Read the model definition and answer for the solid it produces. Units are mm, in the model's axes. A direction names the side the tool comes from. Give positions to 0.01 mm unless a question says otherwise; leave off trailing zeros. Order: outer loops, then holes, each group sorted by start corner. A loop starts at its lowest first (then second) coordinate and runs counter-clockwise, first axis right, second up. Notation, with made-up numbers: M 88,49.5 L 98,49.5 A13 cw 98,59.5 Z; hole C -37.75,63 d9. An arc over 180 degrees is marked long. One line per item, written item: value.
from build123d import *

# Parameters (mm, degrees)
PANEL_W                      = 1000
PANEL_H                      = 300
PANEL_R                      = 117.475
PANEL_R_2                    = 38
PANEL_PLY_DEPTH              = 12
PIZEO_POCKET_CUT_DEPTH       = 3
SKETCH6_R                    = 15
CORD_CUT_DEPTH               = 12
SKETCH7_W                    = 1000
SKETCH7_H                    = 12
HORIZONTAL_HOUSING_CUT_DEPTH = 4
SKETCH8_W                    = 12
SKETCH8_H                    = 276
VERTICAL_HOUSING_CUT_DEPTH   = 4
SKETCH9_R                    = 128.5875
CUT_EXTRUDE1_DEPTH           = 1


with BuildPart() as part:
    # Panel → Panel Ply (new body)
    with BuildSketch(Plane.XY):
        with Locations((500, 150)):
            Rectangle(PANEL_W, PANEL_H)
        with Locations((242, 150)):
            Circle(PANEL_R, mode=Mode.SUBTRACT)
        with Locations((758, 150)):
            Circle(PANEL_R, mode=Mode.SUBTRACT)
        with Locations((68, 150)):
            Circle(PANEL_R_2, mode=Mode.SUBTRACT)
        with Locations(Location((932, 150, 0), (0, 0, 180))):
            Circle(PANEL_R_2, mode=Mode.SUBTRACT)
    extrude(amount=PANEL_PLY_DEPTH)

    # Sketch4 → Pizeo Pocket Cut (cut)
    with BuildSketch(Plane.XY.offset(12)):
        with BuildLine():
            Line((32, 194), (104, 194))
            ThreePointArc((104, 194), (109.656854249, 191.656854249), (112, 186))
            Line((112, 186), (112, 114))
            ThreePointArc((112, 114), (109.656854249, 108.343145751), (104, 106))
            Line((104, 106), (32, 106))
            ThreePointArc((32, 106), (26.343145751, 108.343145751), (24, 114))
            Line((24, 114), (24, 186))
            ThreePointArc((24, 186), (26.343145751, 191.656854249), (32, 194))
        make_face()
        with BuildLine():
            Line((968, 106), (896, 106))
            ThreePointArc((896, 106), (890.343145751, 108.343145751), (888, 114))
            Line((888, 114), (888, 186))
            ThreePointArc((888, 186), (890.343145751, 191.656854249), (896, 194))
            Line((896, 194), (968, 194))
            ThreePointArc((968, 194), (973.656854249, 191.656854249), (976, 186))
            Line((976, 186), (976, 114))
            ThreePointArc((976, 114), (973.656854249, 108.343145751), (968, 106))
        make_face()
    extrude(amount=-PIZEO_POCKET_CUT_DEPTH, mode=Mode.SUBTRACT)

    # Sketch6 → Cord Cut (cut)
    with BuildSketch(Plane.XY.offset(12)):
        with Locations((500, 255)):
            Circle(SKETCH6_R)
    extrude(amount=-CORD_CUT_DEPTH, mode=Mode.SUBTRACT)

    # Sketch7 → Horizontal Housing Cut (cut)
    with BuildSketch(Plane.XY.offset(12)):
        with Locations((500, 294)):
            Rectangle(SKETCH7_W, SKETCH7_H)
        with Locations((500, 6)):
            Rectangle(SKETCH7_W, SKETCH7_H)
    extrude(amount=-HORIZONTAL_HOUSING_CUT_DEPTH, mode=Mode.SUBTRACT)

    # Sketch8 → Vertical Housing Cut (cut)
    with BuildSketch(Plane.XY.offset(12)):
        with Locations((6, 150)):
            Rectangle(SKETCH8_W, SKETCH8_H)
        with Locations((994, 150)):
            Rectangle(SKETCH8_W, SKETCH8_H)
        with Locations((411, 150)):
            Rectangle(SKETCH8_W, SKETCH8_H)
        with Locations((589, 150)):
            Rectangle(SKETCH8_W, SKETCH8_H)
    extrude(amount=-VERTICAL_HOUSING_CUT_DEPTH, mode=Mode.SUBTRACT)

    # Sketch9 → Cut-Extrude1 (cut)
    with BuildSketch(Plane.XY.offset(12)):
        with Locations((242, 150)):
            Circle(SKETCH9_R)
        with Locations(Location((758, 150, 0), (0, 0, 180))):
            Circle(SKETCH9_R)
    extrude(amount=-CUT_EXTRUDE1_DEPTH, mode=Mode.SUBTRACT)


solid = part.part
1) Find section A-A, the plane x = 500. Write down the section's boundary in (y, z), plus the area to 3 significant figures.
Reported:
outline: M 0,0 L 240,0 L 240,12 L 12,12 L 12,8 L 0,8 Z; M 270,0 L 300,0 L 300,8 L 288,8 L 288,12 L 270,12 Z
area: 3,140 mm^2
2) Find section C-C, the plane y = 223. Count the separate pieces of the cut face and the enclosed holes in it, plus the area to 3 significant figures.
Reported:
separate pieces: 3
enclosed holes: 0
area: 7,330 mm^2
3) Determine the mould class of faces 3 (the face through (493, 152, 0)), 4 (the face through (139.957, 71.757, 11.507)) for opening direction X: +X half, -X half, draft (parallel to the pull), parting line (faces both ways), or undercut.
Reported:
face 3: draft
face 4: undercut
4) Find section B-B, the plane z = 4.25. Write down the section's boundary in (x, y) (3 decimals).
Reported:
outline: M 0,0 L 1000,0 L 1000,300 L 0,300 Z; hole C 68,150 d76; hole C 242,150 d234.95; hole C 500,255 d30; hole C 758,150 d234.95; hole C 932,150 d76
5) Each of these flat-tipped pins is pushed along its axis until it touches: pin 1 Ø2 at (x, z) = (461.5, 10.5) entering from -Y; pin 2 Ø1.5 at (y, z) = (135.5, 10) entering from -X; pin 3 Ø2 at (y, z) = (137, 9.5) entering from +X; pin 4 Ø24 at (x, y) = (500, 255) entering from +Z. Where does it stop, or does it pass through?
Reported:
pin 1: stops at y = 12
pin 2: stops at x = 12
pin 3: stops at x = 988
pin 4: passes through
6) Which of the six approach directions +Z, -Z, +X, -X, +Y, -Y give full straight-line access (tool end or side, diameter ignored) to faces 1 (the face through (639.22, 199.25, 11.51)), 2 (the face through (640.64, 155.17, 5.42))?
Reported:
face 1: +Z
face 2: +Z, -Z
7) Consider probe 1 along X at (y, z) = (146.5, 6); probe 2 along Y at (x, z) = (932, 4.75); probe 3 along Y at (x, z) = (758, 11.3). Determine where each line is inside the solid, lowest interval first.
Reported:
probe 1: x = 0 to 30.16, 105.84 to 124.58, 359.42 to 640.58, 875.42 to 894.16, 969.84 to 1000
probe 2: y = 0 to 112, 188 to 300
probe 3: y = 12 to 21.41, 278.59 to 288
